from build123d import *
from build123d.topology import SkipClean

# Parameters (mm, degrees)
SKETCH1_W           = 100
SKETCH1_H           = 22.5
BOSS_EXTRUDE1_DEPTH = 55.5
CUT_EXTRUDE1_DEPTH  = 79.016023995
CUT_EXTRUDE2_DEPTH  = 73.059409747
CUT_EXTRUDE3_DEPTH  = 73.059409747
SKETCH6_R           = 12
SKETCH6_R_2         = 10
BOSS_EXTRUDE2_DEPTH = 5
BOSS_EXTRUDE3_START = 19
SKETCH7_R           = 19.927383843
SKETCH7_R_2         = 10
BOSS_EXTRUDE3_DEPTH = 19
BOSS_EXTRUDE5_START = 10
SKETCH9_R           = 32.155692567
SKETCH9_R_2         = 10
BOSS_EXTRUDE5_DEPTH = 10


with BuildPart() as part:
    # Sketch1 → Boss-Extrude1 (new body)
    with BuildSketch(Plane(origin=(0, 0, 0), x_dir=(0, 1, 0), z_dir=(0, 0, 1))):
        with Locations((0, -11.25)):
            Rectangle(SKETCH1_W, SKETCH1_H)
    extrude(amount=BOSS_EXTRUDE1_DEPTH)

    # Sketch2 → Cut-Extrude1 (cut, through all)
    with BuildSketch(Plane.YZ.offset(22.5)):
        with BuildLine():
            Line((-50, 8.742021972), (-24, 8.742021972))
            Line((-24, 8.742021972), (-24, 14.574278418))
            ThreePointArc((-24, 14.574278418), (-27.5, 28), (-24, 41.425721582))
            Line((-24, 41.425721582), (-24, 55.5))
            Line((-24, 55.5), (-50, 55.5))
            Line((-50, 55.5), (-50, 8.742021972))
        make_face()
        with BuildLine():
            ThreePointArc((-24, 41.425721582), (-27.5, 28), (-24, 14.574278418))
            Line((-24, 14.574278418), (-24, 27.75))
            add(Edge.make_bspline(
                [(-24, 28.630883492), (-24.003292455, 28.193991063), (-24, 27.75)],
                knots=[0.983572463, 0.983572463, 0.983572463, 1, 1, 1], degree=2))
            Line((-24, 28.630883492), (-24, 41.425721582))
        make_face()
        with BuildLine():
            ThreePointArc((-15.102725788, 50.981681265), (-20.126720607, 46.73940014), (-24, 41.425721582))
            Line((-24, 41.425721582), (-24, 28.630883492))
            add(Edge.make_bspline(
                [(-15.102725788, 50.981681265), (-23.880610505, 44.473278164), (-24, 28.630883492)],
                knots=[0.387884574, 0.387884574, 0.387884574, 0.983572463, 0.983572463, 0.983572463], degree=2))
        make_face()
        with BuildLine():
            Line((-24, 55.5), (-24, 41.425721582))
            ThreePointArc((-24, 41.425721582), (-20.126720607, 46.73940014), (-15.102725788, 50.981681265))
            add(Edge.make_bspline(
                [(-5.719329936, 54.898685192), (-11.246534385, 53.840872164), (-15.102725788, 50.981681265)],
                knots=[0.126194361, 0.126194361, 0.126194361, 0.387884574, 0.387884574, 0.387884574], degree=2))
            ThreePointArc((-5.719329936, 54.898685192), (-2.875426682, 55.349258151), (0, 55.5))
            Line((0, 55.5), (-24, 55.5))
        make_face()
        with BuildLine():
            ThreePointArc((0, 38), (-10, 28), (0, 18))
            Line((0, 18), (0, 38))
        make_face()
        with BuildLine():
            Line((0, 38), (0, 18))
            ThreePointArc((0, 18), (7.071067812, 20.928932188), (10, 28))
            ThreePointArc((10, 28), (7.071067812, 35.071067812), (0, 38))
        make_face()
        with BuildLine():
            Line((24, 55.5), (0, 55.5))
            ThreePointArc((0, 55.5), (2.875426682, 55.349258151), (5.719329936, 54.898685192))
            add(Edge.make_bspline(
                [(5.719329936, 54.898685192), (11.246534385, 53.840872164), (15.102725788, 50.981681265)],
                knots=[0.126194361, 0.126194361, 0.126194361, 0.387884574, 0.387884574, 0.387884574], degree=2))
            ThreePointArc((15.102725788, 50.981681265), (20.126720607, 46.73940014), (24, 41.425721582))
            Line((24, 41.425721582), (24, 55.5))
        make_face()
        with BuildLine():
            Line((24, 14.574278418), (24, 8.742021972))
            Line((24, 8.742021972), (50, 8.742021972))
            Line((50, 8.742021972), (50, 14.574278418))
            Line((50, 14.574278418), (50, 55.5))
            Line((50, 55.5), (24, 55.5))
            Line((24, 55.5), (24, 41.425721582))
            ThreePointArc((24, 41.425721582), (26.610618181, 34.937218463), (27.5, 28))
            ThreePointArc((27.5, 28), (26.610618181, 21.062781537), (24, 14.574278418))
        make_face()
        with BuildLine():
            Line((24, 27.75), (24, 14.574278418))
            ThreePointArc((24, 14.574278418), (26.610618181, 21.062781537), (27.5, 28))
            ThreePointArc((27.5, 28), (26.610618181, 34.937218463), (24, 41.425721582))
            Line((24, 41.425721582), (24, 28.630883492))
            add(Edge.make_bspline(
                [(24, 28.630883492), (24.003292455, 28.193991063), (24, 27.75)],
                knots=[0.983572463, 0.983572463, 0.983572463, 1, 1, 1], degree=2))
        make_face()
        with BuildLine():
            ThreePointArc((24, 41.425721582), (20.126720607, 46.73940014), (15.102725788, 50.981681265))
            add(Edge.make_bspline(
                [(15.102725788, 50.981681265), (23.880610505, 44.473278164), (24, 28.630883492)],
                knots=[0.387884574, 0.387884574, 0.387884574, 0.983572463, 0.983572463, 0.983572463], degree=2))
            Line((24, 28.630883492), (24, 41.425721582))
        make_face()
    extrude(amount=-CUT_EXTRUDE1_DEPTH, mode=Mode.SUBTRACT)

    # Sketch3 → Cut-Extrude2 (cut, through all)
    with BuildSketch(Plane.XY.offset(8.742021972)):
        with BuildLine():
            ThreePointArc((16.25, 37), (15.797494838, 39.078530898), (14.521883722, 40.780843412))
            Line((14.521883722, 40.780843412), (7.978116278, 33.219156588))
            ThreePointArc((7.978116278, 33.219156588), (13.328530898, 32.452505162), (16.25, 37))
        make_face()
        with BuildLine():
            Line((7.978116278, 33.219156588), (14.521883722, 40.780843412))
            ThreePointArc((14.521883722, 40.780843412), (7.469156588, 40.271883722), (7.978116278, 33.219156588))
        make_face()
    extrude(amount=-CUT_EXTRUDE2_DEPTH, mode=Mode.SUBTRACT)

    # Sketch5 → Cut-Extrude3 (cut, through all)
    with BuildSketch(Plane.XY.offset(8.742021972)):
        with BuildLine():
            ThreePointArc((16.248437988, -37), (13.32788156, -32.45392581), (7.979138422, -33.220337732))
            Line((7.979138422, -33.220337732), (14.520861578, -40.779662268))
            ThreePointArc((14.520861578, -40.779662268), (15.79607419, -39.07788156), (16.248437988, -37))
        make_face()
        with BuildLine():
            Line((14.520861578, -40.779662268), (7.979138422, -33.220337732))
            ThreePointArc((7.979138422, -33.220337732), (7.470337732, -40.270861578), (14.520861578, -40.779662268))
        make_face()
    extrude(amount=-CUT_EXTRUDE3_DEPTH, mode=Mode.SUBTRACT)

    # Sketch6 → Boss-Extrude2 (add)
    with SkipClean():  # the faces are left unmerged after this step: merging them gives an invalid solid
        with BuildSketch(Plane(origin=(0, 0, 0), x_dir=(0, -1, 0), z_dir=(-1, 0, 0))):
            with Locations(Location((0, 28, 0), (0, 0, 270))):
                Circle(SKETCH6_R)
            with Locations(Location((0, 28, 0), (0, 0, 270))):
                Circle(SKETCH6_R_2, mode=Mode.SUBTRACT)
        extrude(amount=BOSS_EXTRUDE2_DEPTH)

    # Sketch7 → Boss-Extrude3 (add)
    with SkipClean():  # the faces are left unmerged after this step: merging them gives an invalid solid
        with BuildSketch(Plane.YZ.offset(22.5).offset(BOSS_EXTRUDE3_START)):
            with Locations(Location((0, 28, 0), (0, 0, 270))):
                Circle(SKETCH7_R)
            with Locations(Location((0, 28, 0), (0, 0, 270))):
                Circle(SKETCH7_R_2, mode=Mode.SUBTRACT)
        extrude(amount=-BOSS_EXTRUDE3_DEPTH)

    # Sketch9 → Boss-Extrude5 (add)
    with SkipClean():  # the faces are left unmerged after this step: merging them gives an invalid solid
        with BuildSketch(Plane.YZ.offset(41.5).offset(BOSS_EXTRUDE5_START)):
            with Locations(Location((0, 28, 0), (0, 0, 270))):
                Circle(SKETCH9_R)
            with Locations(Location((0, 28, 0), (0, 0, 270))):
                Circle(SKETCH9_R_2, mode=Mode.SUBTRACT)
        extrude(amount=-BOSS_EXTRUDE5_DEPTH)


solid = part.part
Can you work these out from the model? Positions are in its coordinate system, mm. A direction names the side the tool comes from. Give positions to 0.01 mm unless a question says otherwise; leave off trailing zeros. Order: outer loops, then holes, each group sorted by start corner. A loop starts at its lowest first (then second) coordinate and runs counter-clockwise, first axis right, second up. Notation, with made-up numbers: M -5,25.25 L 17,25.25 A5 ccw 17,31.25 Z; hole C 70,-25.5 d11. An arc over 180 degrees is marked long. Use one line per item in the form item = value. Start each with the question number.
Item 1: If we section it at B-B (y = -35): Write out the boundary of the cut face in (x, z).
Item 2: Will these pins go through, and if not, where does the flat tip stop? pin 1 Ø5 at (x, y) = (1, 9) entering from -Z; pin 2 Ø15 at (x, z) = (8.5, 18.5) entering from +Y; pin 3 Ø12 at (x, z) = (45.5, 14.5) entering from -Y.
Item 3: If I drill on line 1 along Y through (x, z) = (-3.3, 28); line 2 along X through (y, z) = (13.5, 9); line 3 along Y through (x, z) = (49.25, 28), over which ranges is the centre line in solid material (lowest first)?
Item 4: We'd pull the mould along X, two halves only. Please class faces 4 (the cylindrical face through (46.57, 9.66, -2.67)), 5 (the cylindrical face through (32.13, -12.13, 43.81)), 6 (the flat face through (-5, -9, 33)): +X half, -X half, draft (parallel to the pull), parting line (faces both ways), or undercut.
Item 5: For faces 1 (the flat face through (22.5, 0, 7)), 2 (the flat face through (16.4, 36.8, 8.742)), 3 (the flat face through (11, -24, 18)), which set-ups out of +Z, -Z, +X, -X, +Y, -Y let a thin tool reach every point of the face, with its end or its side?
Item 6: If we section it at A-A (x = 11.25): State how many separate pieces and enclosed holes the cut face has, then the cut area to 3 significant figures.
Item 7: If we section it at C-C (x = 45): Write out the boundary of the cut face in (y, z).
Outcome:
q1.outline = M 0,0 L 6.67,0 L 6.67,8.74 L 0,8.74 Z; M 15.83,0 L 22.5,0 L 22.5,8.74 L 15.83,8.74 Z
q2.pin_1 = 0
q2.pin_2 = 24
q2.pin_3 = -31.27
q3.line_1 = -12 to -10, 10 to 12
q3.line_2 = 0 to 22.5, 41.5 to 51.5
q3.line_3 = -32.16 to -10, 10 to 32.16
q4.face_4 = draft
q4.face_5 = undercut
q4.face_6 = -X half
q5.face_1 = none
q5.face_2 = +Z, -X, +Y
q5.face_3 = +Z, -X, -Y
q6.separate_pieces = 3
q6.enclosed_holes = 1
q6.area = 2,400 mm2
q7.outline = C 0,28 d64.31; hole C 0,28 d20
